Part model, mm, in its own coordinate system. A direction names the side the tool comes from. Give positions to 0.01 mm unless a question says otherwise; leave off trailing zeros. Loops run counter-clockwise (first coordinate to the right, second up) from the corner with the lowest first, then second, coordinate; pieces in that order, holes last. Notation, with made-up numbers: M -25,-26.5 L 1,-26.5 A18 cw 1,5.5 Z; hole C 86.5,4.5 d4. An arc over 180 degrees is marked long. Answer in a Markdown table with one row per item.
from build123d import *

# Parameters (mm, degrees)
F0_R     = 6.35
F1_DEPTH = 254
F2_R     = 2.38125
F3_DEPTH = 12.7
F4_W     = 38.273203
F4_H     = 14.002507
F5_DEPTH = 12.7


with BuildPart() as f1:
    # F0 (on Top) → F1 (new body)
    with BuildSketch(Plane.XY):
        Circle(F0_R)
    extrude(amount=F1_DEPTH)

    # F2 (on Front) → F3 (cut, symmetric)
    with BuildSketch(Plane.XZ):
        with Locations((0, 5.08)):
            Circle(F2_R)
    extrude(amount=F3_DEPTH, both=True, mode=Mode.SUBTRACT)

    # F4 (on face) → F5 (cut)
    with BuildSketch(Plane(origin=(0, 0, 0), x_dir=(1, 0, 0), z_dir=(0, 0, -1))):
        with Locations((-1.712646, 12.081253)):
            Rectangle(F4_W, F4_H)
    extrude(amount=-F5_DEPTH, mode=Mode.SUBTRACT)


solid = f1.part
(1) Saw through at C-C (y = -2.5). Write the cut outline in (x, z), plus the area to 3 significant figures.
Recorded:
| item | result |
|---|---|
| outline | M -5.84,0 L 5.84,0 L 5.84,254 L -5.84,254 Z; hole C 0,5.08 d4.76 |
| area | 2,950 mm^2 |
(2) Saw through at D-D (z = 205.5). Write the cut outline in (x, y), plus the area to 3 significant figures.
Recorded:
| item | result |
|---|---|
| outline | C 0,0 d12.7 |
| area | 127 mm^2 |
(3) Saw through at B-B (z = 5.08). Write the cut outline in (x, y).
Recorded:
| item | result |
|---|---|
| outline | M -3.81,-5.08 L -2.38,-5.08 L -2.38,5.89 A6.35 ccw Z; M 2.38,-5.08 L 3.81,-5.08 A6.35 ccw 2.38,5.89 Z |
(4) Drill centre lines: line 1 along Z through (x, y) = (0, 4); line 2 along X through (y, z) = (-0.25, 5.08); line 3 along Y through (x, z) = (0.25, 31). Where is each one in solid material? Low to high.
Recorded:
| item | result |
|---|---|
| line 1 | z = 0 to 2.7, 7.46 to 254 |
| line 2 | x = -6.35 to -2.38, 2.38 to 6.35 |
| line 3 | y = -6.35 to 6.35 |
(5) Saw through at A-A (x = 0). Write the cut outline in (y, z).
Recorded:
| item | result |
|---|---|
| outline | M -6.35,12.7 L -5.08,12.7 L -5.08,7.46 L 6.35,7.46 L 6.35,254 L -6.35,254 Z; M -5.08,0 L 6.35,0 L 6.35,2.7 L -5.08,2.7 Z |
(6) Pull direction X, two halves, no side cores. Call faces 3 (the face through (0, 0, 254)), 4 (the face through (-0.516, 0.556, 2.755)), 5 (the face through (-0.8, 6.3, 125.2)): +X half, -X half, draft (parallel to the pull), parting line (faces both ways), or undercut.
Recorded:
| item | result |
|---|---|
| face 3 | draft |
| face 4 | undercut |
| face 5 | parting line |
(7) Pin check, flat tips, straight feed: pin 1 Ø1.4 at (x, y) = (1.5, -6) entering from -Z; pin 2 Ø1 at (x, z) = (0.5, 171.5) entering from -Y; pin 3 Ø1.5 at (x, z) = (-4, 44) entering from +Y; pin 4 Ø4 at (x, z) = (0, 5.5) entering from -Y. Stop position of each tip, or through.
Recorded:
| item | result |
|---|---|
| pin 1 | stops at z = 12.7 |
| pin 2 | stops at y = -6.35 |
| pin 3 | stops at y = 5.46 |
| pin 4 | stops at y = -5.08 |
(8) Which spindle directions (+Z, -Z, +X, -X, +Y, -Y) get a long thin tool onto all of the face, cutting with end or side? Do faces 1 (the face through (0, -5.08, 8)), 2 (the face through (0, 1, 0)). Say none if no direction does.
Recorded:
| item | result |
|---|---|
| face 1 | -Z, +X, -X, -Y |
| face 2 | -Z, +X, -X, +Y, -Y |
